The model under review builds one solid part; all positions refer to its coordinate system, in mm. Face numbers are marked on the shaded views. A direction names the side the tool comes from. Give positions to 0.01 mm unless a question says otherwise; leave off trailing zeros. Loops run counter-clockwise (first coordinate to the right, second up) from the corner with the lowest first, then second, coordinate; pieces in that order, holes last. Notation, with made-up numbers: M 35.5,83.25 L 66.5,83.25 A6 cw 66.5,92.25 Z; hole C 3.25,54.25 d8. An arc over 180 degrees is marked long. Write item = value, one per line. Start each with the question number.
1. For the marked faces 1, 2, 3, 4 and 5, list the 3-axis set-ups (+Z, -Z, +X, -X, +Y, -Y) from which the entire face can be reached by the end or side of a thin tool; tool diameter is ignored.
2. We need section D-D on y = -30.5. Give the boundary of the cut face in (x, z).
3. We need section A-A on z = 2.25. Give the boundary of the cut face in (x, y).
4. We need section B-B on y = -50. Give the boundary of the cut face in (x, z), then the cut area to 3 significant figures.
5. Wall thickness on line 1 along Y through (x, z) = (6, 9.5); line 2 along X through (y, z) = (-27.5, 9.5); line 3 along Z through (x, y) = (23, -29.25): over which ranges is each line inside the solid? List them lowest first. Write a range as from..to.
6. We need section C-C on x = 6. Give the boundary of the cut face in (y, z), then the cut area to 3 significant figures.
7. For pin 1 (1 mm diameter, centred on x = 30.5, z = 1.5, fed in from -Y); pin 2 (6.5 mm diameter, centred on x = 9.5, y = -50, fed in from +Z); pin 3 (1.5 mm diameter, centred on y = -48.5, z = 2.5, fed in from +X), all flat-tipped, find the tip position at first contact; note any pin that passes through.
from build123d import *

# Parameters (mm, degrees)
BOX001_W     = 14
BOX001_H     = 10
BOX001_DEPTH = 11
BOX002_W     = 8.3
BOX002_H     = 6
BOX002_DEPTH = 3
BOX_W        = 42
BOX_H        = 24.5
BOX_DEPTH    = 1.6


with BuildPart() as cube001:
    # Box001 → Box001 (new body)
    with BuildSketch(Plane(origin=(1, 16, 1.6), x_dir=(1, 0, 0), z_dir=(0, 0, 1))):
        with Locations((7, 5)):
            Rectangle(BOX001_W, BOX001_H)
    extrude(amount=BOX001_DEPTH)


with BuildPart() as cube002:
    # Box002 → Box002 (new body)
    with BuildSketch(Plane(origin=(5, -1, 1.6), x_dir=(1, 0, 0), z_dir=(0, 0, 1))):
        with Locations((4.15, 3)):
            Rectangle(BOX002_W, BOX002_H)
    extrude(amount=BOX002_DEPTH)


with BuildPart() as obj1:
    # Box → Box (new body)
    with BuildSketch(Plane.XY):
        with Locations((21, 12.25)):
            Rectangle(BOX_W, BOX_H)
    extrude(amount=BOX_DEPTH)

    # Fusion: union Cube001, Cube002
    add(cube001.part)
    add(cube002.part)


with BuildPart() as obj1_1:
    # Fusion placement: moved
    add(obj1.part.moved(Location((0, -51, 0))))


solid = obj1_1.part
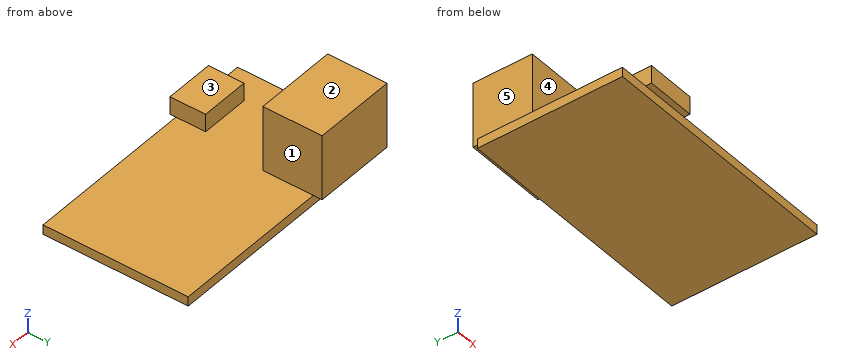
Final values:
q1.face_1 = +Z, +X, +Y, -Y
q1.face_2 = +Z, +X, -X, +Y, -Y
q1.face_3 = +Z, +X, -X, -Y
q1.face_4 = +Z, +X, -X
q1.face_5 = +Z, -X, +Y, -Y
q2.outline = M 0,0 L 42,0 L 42,1.6 L 15,1.6 L 15,12.6 L 1,12.6 L 1,1.6 L 0,1.6 Z
q3.outline = M 1,-35 L 15,-35 L 15,-25 L 1,-25 Z; M 5,-52 L 13.3,-52 L 13.3,-46 L 5,-46 Z
q4.outline = M 0,0 L 42,0 L 42,1.6 L 13.3,1.6 L 13.3,4.6 L 5,4.6 L 5,1.6 L 0,1.6 Z
q4.area = 92.1 mm²
q5.line_1 = -35..-25
q5.line_2 = 1..15
q5.line_3 = 0..1.6
q6.outline = M -52,1.6 L -51,1.6 L -51,0 L -26.5,0 L -26.5,1.6 L -25,1.6 L -25,12.6 L -35,12.6 L -35,1.6 L -46,1.6 L -46,4.6 L -52,4.6 Z
q6.area = 167 mm²
q7.pin_1 = -51
q7.pin_2 = 4.6
q7.pin_3 = 13.3
